Build history of the part. All positions in model axes, mm. A direction names the side the tool comes from. Round coordinates to 2 decimals unless told otherwise and drop trailing zeros. Write each loop counter-clockwise with the first axis right and the second up, starting at its lowest first coordinate (ties: lowest second). Pieces come first, ordered by that corner, then holes.
1) Saw through at C-C (y = 0.6). State how many separate pieces and enclosed holes the cut face has, plus the area to 3 significant figures.
2) Wall check: probe 1 along X at (y, z) = (2.25, -150); probe 2 along X at (y, z) = (1.1, -32.5); probe 3 along X at (y, z) = (2, -47). Give the ranges that are in metal, low to high.
3) Saw through at A-A (x = 82.5). Write the cut outline in (y, z), plus the area to 3 significant figures.
4) Pull direction Z, two halves, no side cores. Call faces 1 (the flat face through (99, 3, -87)), 2 (the cylindrical face through (50.138, 1.521, -61.056)), 3 (the flat face through (103.879, 1.521, -112.284)): +Z half, -Z half, draft (parallel to the pull), parting line (faces both ways), or undercut.
5) Which spindle directions (+Z, -Z, +X, -X, +Y, -Y) get a long thin tool onto all of the face, cutting with end or side? Do faces 4 (the flat face through (99, 0, -87)), 5 (the flat face through (106.12, 1.52, -108.96)). Say none if no direction does.
6) Saw through at B-B (z = -41.5). Write the cut outline in (x, y), plus the area to 3 significant figures.
from build123d import *

# Parameters (mm, degrees)
SKETCH1_W                = 200
SKETCH1_H                = 200
BOSS_EXTRUDE1_DEPTH      = 3
SKETCH2_R                = 13
SKETCH2_R_2              = 15
CUT_EXTRUDE1_DEPTH       = 283.85862193
M3_CLEARANCE_HOLE1_D     = 3.4
M3_CLEARANCE_HOLE2_D     = 3.4
SKETCH8_W                = 200
SKETCH8_H                = 30
BOSS_EXTRUDE2_DEPTH      = 3
M4_CLEARANCE_HOLE1_D     = 4.5
M4_CLEARANCE_HOLE1_DEPTH = 7
M4_CLEARANCE_HOLE1_TIP   = 1.351936393


with BuildPart() as part:
    # Sketch1 → Boss-Extrude1 (new body)
    with BuildSketch(Plane(origin=(0, 0, 0), x_dir=(1, 0, 0), z_dir=(0, 1, 0))):
        with Locations((100, 100)):
            Rectangle(SKETCH1_W, SKETCH1_H)
    extrude(amount=BOSS_EXTRUDE1_DEPTH)

    # Sketch2 → Cut-Extrude1 (cut, through all)
    with BuildSketch(Plane(origin=(0, 3, 0), x_dir=(1, 0, 0), z_dir=(0, 1, 0))):
        with Locations(Location((90, 136.602540378, 0), (0, 0, 270))):
            Circle(SKETCH2_R)
        with Locations(Location((140, 50, 0), (0, 0, 270))):
            Circle(SKETCH2_R)
        with Locations(Location((40, 50, 0), (0, 0, 270))):
            Circle(SKETCH2_R_2)
        with BuildLine():
            Line((95.339745962, 107.353829072), (112.660254038, 117.353829072))
            ThreePointArc((112.660254038, 117.353829072), (115.392304845, 116.621778265), (114.660254038, 113.889727457))
            Line((114.660254038, 113.889727457), (97.339745962, 103.889727457))
            ThreePointArc((97.339745962, 103.889727457), (94.607695155, 104.621778265), (95.339745962, 107.353829072))
        make_face()
    extrude(amount=-CUT_EXTRUDE1_DEPTH, mode=Mode.SUBTRACT)

    # M3 Clearance Hole1 (through all)
    with Locations(Plane(origin=(0, 3, 0), x_dir=(1, 0, 0), z_dir=(0, 1, 0))):
        with Locations((140, 67.5), (122.5, 50), (157.5, 50), (140, 32.5), (90, 119.102540378), (72.5, 136.602540378), (107.5, 136.602540378), (90, 154.102540378)):
            Hole(M3_CLEARANCE_HOLE1_D / 2)

    # M3 Clearance Hole2 (through all)
    with Locations(Plane(origin=(0, 3, 0), x_dir=(1, 0, 0), z_dir=(0, 1, 0))):
        with Locations((16.184301396, 63.75), (63.815698604, 36.25)):
            Hole(M3_CLEARANCE_HOLE2_D / 2)

    # Sketch8 → Boss-Extrude2 (add)
    with BuildSketch(Plane(origin=(0, 3, 0), x_dir=(1, 0, 0), z_dir=(0, 1, 0))):
        with Locations((100, -15)):
            Rectangle(SKETCH8_W, SKETCH8_H)
    extrude(amount=-BOSS_EXTRUDE2_DEPTH)

    # M4 Clearance Hole1
    with Locations(Plane(origin=(0, 3, 0), x_dir=(1, 0, 0), z_dir=(0, 1, 0))):
        with Locations((30, 0), (30, 150), (130, 150)):
            Hole(M4_CLEARANCE_HOLE1_D / 2, depth=M4_CLEARANCE_HOLE1_DEPTH)
            with Locations((0, 0, -(M4_CLEARANCE_HOLE1_DEPTH + M4_CLEARANCE_HOLE1_TIP / 2))):  # 118° drill point
                Cone(0, M4_CLEARANCE_HOLE1_D / 2, M4_CLEARANCE_HOLE1_TIP, mode=Mode.SUBTRACT)


solid = part.part
Evaluation:
1. separate pieces: 1
1. enclosed holes: 17
1. area: 44,000 mm2
2. probe 1: x = 0 to 27.75, 32.25 to 127.75, 132.25 to 200
2. probe 2: x = 0 to 138.3, 141.7 to 200
2. probe 3: x = 0 to 25.3, 54.7 to 127.35, 152.65 to 200
3. outline: (0, -200) - (3, -200) - (3, -147.22) - (0, -147.22) - close; (0, -125.98) - (3, -125.98) - (3, 30) - (0, 30) - close
3. area: 626 mm2
4. face 1: draft
4. face 2: undercut
4. face 3: undercut
5. face 4: +Z, -Z, +X, -X, -Y
5. face 5: +Y, -Y
6. outline: (0, 0) - (27.64, 0) - (27.64, 3) - (0, 3) - close; (52.36, 0) - (130.16, 0) - (130.16, 3) - (52.36, 3) - close; (149.84, 0) - (200, 0) - (200, 3) - (149.84, 3) - close
6. area: 467 mm2
